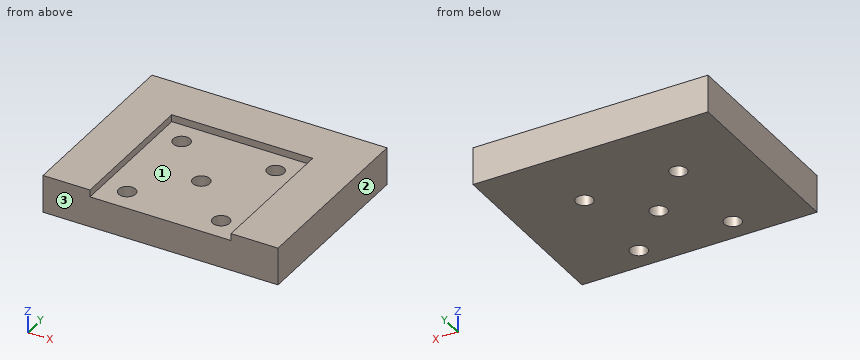
```python
from build123d import *
from build123d import SkipClean  # not in build123d's __all__

# Parameters (mm, degrees)
F0_R      = 2.85
F0_R_2    = 11
F1_DEPTH  = 40
F2_W      = 30
F2_H      = 30
F3_DEPTH  = 55
F5_DEPTH  = 30
F6_DEPTH  = 40.001
F7_DEPTH  = 40.001
F8_R      = 1.8
F9_DEPTH  = 11.5
F10_DEPTH = 13
F11_DEPTH = 5


with BuildPart() as f1:
    # F0 (on Front) → F1 (new body)
    with BuildSketch(Plane.XZ):
        with BuildLine():
            Line((15, 28.25), (-15, 28.25))
            ThreePointArc((-15, 28.25), (-22.0710678119, 25.3210678119), (-25, 18.25))
            Line((-25, 18.25), (-25, -38.25))
            Line((-25, -38.25), (25, -38.25))
            Line((25, -38.25), (25, 18.25))
            ThreePointArc((25, 18.25), (22.0710678119, 25.3210678119), (15, 28.25))
        make_face()
        with Locations((0, -18.25)):
            Circle(F0_R, mode=Mode.SUBTRACT)
        Circle(F0_R_2, mode=Mode.SUBTRACT)
        with Locations((0, 18.25)):
            Circle(F0_R, mode=Mode.SUBTRACT)
    extrude(amount=F1_DEPTH)

    # F2 (on face) → F3 (cut)
    with BuildSketch(Plane.XY.offset(28.25)):
        with Locations((0, -25)):
            Rectangle(F2_W, F2_H)
    extrude(amount=-F3_DEPTH, mode=Mode.SUBTRACT)

    # F4 (on face) → F5 (join, through all)
    with BuildSketch(Plane.XZ.offset(40)):
        with BuildLine():
            Line((-15, 17.2291616466), (-15, 19.972135955))
            ThreePointArc((-15, 19.972135955), (-20, 15.5), (-15, 11.027864045))
            Line((-15, 11.027864045), (-15, 13.7708383534))
            ThreePointArc((-15, 13.7708383534), (-17.3, 15.5), (-15, 17.2291616466))
        make_face()
        with BuildLine():
            Line((-15, -17.2291616466), (-15, -19.972135955))
            ThreePointArc((-15, -19.972135955), (-12.1458980338, -18.5), (-11, -15.5))
            ThreePointArc((-11, -15.5), (-12.1458980338, -12.5), (-15, -11.027864045))
            Line((-15, -11.027864045), (-15, -13.7708383534))
            ThreePointArc((-15, -13.7708383534), (-14.061250543, -14.4183346174), (-13.7, -15.5))
            ThreePointArc((-13.7, -15.5), (-14.061250543, -16.5816653826), (-15, -17.2291616466))
        make_face()
        with BuildLine():
            ThreePointArc((20, -15.5), (18.5, -12.1458980338), (15, -11.027864045))
            Line((15, -11.027864045), (15, -13.7708383534))
            ThreePointArc((15, -13.7708383534), (16.5816653826, -14.061250543), (17.3, -15.5))
            ThreePointArc((17.3, -15.5), (16.5816653826, -16.938749457), (15, -17.2291616466))
            Line((15, -17.2291616466), (15, -19.972135955))
            ThreePointArc((15, -19.972135955), (18.5, -18.8541019662), (20, -15.5))
        make_face()
        with BuildLine():
            Line((15, 17.2291616466), (15, 19.972135955))
            ThreePointArc((15, 19.972135955), (11, 15.5), (15, 11.027864045))
            Line((15, 11.027864045), (15, 13.7708383534))
            ThreePointArc((15, 13.7708383534), (13.7, 15.5), (15, 17.2291616466))
        make_face()
    extrude(amount=-F5_DEPTH)

    # F4 (on face) → F6 (cut, through all)
    with BuildSketch(Plane.XZ.offset(40)):
        with BuildLine():
            ThreePointArc((-13.7, 15.5), (-14.061250543, 16.5816653826), (-15, 17.2291616466))
            Line((-15, 17.2291616466), (-15, 13.7708383534))
            ThreePointArc((-15, 13.7708383534), (-14.061250543, 14.4183346174), (-13.7, 15.5))
        make_face()
        with BuildLine():
            ThreePointArc((17.3, 15.5), (16.5816653826, 16.938749457), (15, 17.2291616466))
            Line((15, 17.2291616466), (15, 13.7708383534))
            ThreePointArc((15, 13.7708383534), (16.5816653826, 14.061250543), (17.3, 15.5))
        make_face()
        with BuildLine():
            Line((15, -17.2291616466), (15, -13.7708383534))
            ThreePointArc((15, -13.7708383534), (13.7, -15.5), (15, -17.2291616466))
        make_face()
        with BuildLine():
            ThreePointArc((-15, -13.7708383534), (-17.3, -15.5), (-15, -17.2291616466))
            Line((-15, -17.2291616466), (-15, -13.7708383534))
        make_face()
    with SkipClean():  # cleaning this boolean's faces spoils the solid; the shape is the same uncleaned
        extrude(amount=-F6_DEPTH, mode=Mode.SUBTRACT)

    # F4 (on face) → F7 (cut, through all)
    with BuildSketch(Plane.XZ.offset(40)):
        with BuildLine():
            Line((-15, 13.7708383534), (-15, 17.2291616466))
            ThreePointArc((-15, 17.2291616466), (-17.3, 15.5), (-15, 13.7708383534))
        make_face()
        with BuildLine():
            Line((15, 13.7708383534), (15, 17.2291616466))
            ThreePointArc((15, 17.2291616466), (13.7, 15.5), (15, 13.7708383534))
        make_face()
        with BuildLine():
            Line((-15, -13.7708383534), (-15, -17.2291616466))
            ThreePointArc((-15, -17.2291616466), (-14.061250543, -16.5816653826), (-13.7, -15.5))
            ThreePointArc((-13.7, -15.5), (-14.061250543, -14.4183346174), (-15, -13.7708383534))
        make_face()
        with BuildLine():
            ThreePointArc((17.3, -15.5), (16.5816653826, -14.061250543), (15, -13.7708383534))
            Line((15, -13.7708383534), (15, -17.2291616466))
            ThreePointArc((15, -17.2291616466), (16.5816653826, -16.938749457), (17.3, -15.5))
        make_face()
    with SkipClean():  # cleaning this boolean's faces spoils the solid; the shape is the same uncleaned
        extrude(amount=-F7_DEPTH, mode=Mode.SUBTRACT)

    # F8 (on face) → F9 (cut, through all)
    with BuildSketch(Plane.XY.offset(-26.75)):
        with Locations((-10, -15)):
            Circle(F8_R)
        with Locations((10, -15)):
            Circle(F8_R)
        with Locations((-10, -35)):
            Circle(F8_R)
        with Locations((10, -35)):
            Circle(F8_R)
        with Locations((0, -25)):
            Circle(F8_R)
    extrude(amount=-F9_DEPTH, mode=Mode.SUBTRACT)

    # F10 (intersect): a face of the model
    f10_faces = [f1.faces().sort_by_distance(p)[0] for p in [
        (0, -19.8694432325, -38.25),
    ]]
    extrude(f10_faces, amount=-F10_DEPTH, mode=Mode.INTERSECT)

    # F11 (cut): a face of the model
    f11_faces = [f1.faces().sort_by_distance(p)[0] for p in [
        (0, -19.8694432325, -38.25),
    ]]
    extrude(f11_faces, amount=-F11_DEPTH, mode=Mode.SUBTRACT)


solid = f1.part
```
Part model, mm, in its own coordinate system. Face numbers are marked on the shaded views. Round coordinates to 2 decimals unless told otherwise and drop trailing zeros. Write each loop counter-clockwise with the first axis right and the second up, starting at its lowest first coordinate (ties: lowest second). Pieces come first, ordered by that corner, then holes. Notation, with made-up numbers: M -20,-37.75 L 30,-37.75 A9 ccw 30,-22.75 Z; hole C -38.5,-14 d11. An arc over 180 degrees is marked long. Answer as CSV lines item,"result". Start each with the question number.
1) Drop flat-ended pins along their axis: pin 1 (4.5 mm diameter, centred on x = 10, y = -35, fed in from +Z); pin 2 (2 mm diameter, centred on x = 10, y = -15, fed in from -Z). Give the stop position or say it passes through.
2) Band-saw the part on C-C (z = -31.25). List the corners of the cut face in (x, y).
3) Band-saw the part on D-D (x = 0). List the corners of the cut face in (y, z).
4) Band-saw the part on B-B (y = -25). List the corners of the cut face in (x, z).
5) Band-saw the part on A-A (x = -10). List the corners of the cut face in (y, z), then the cut area to 3 significant figures.
6) Mould opens along X. For the marked faces 1, 2 and 3 say: +X half, -X half, draft (parallel to the pull), parting line (faces both ways), or undercut.
7) Drill centre lines: L1, parallel to Y at x = 10, z = -28.75; L2, parallel to Y at x = 0, z = -30.5; L3, parallel to X at y = -12.5, z = -25.75. Where is each one in solid material? Low to high.
Worked out:
1,pin 1,"z = -26.75"
1,pin 2,"through"
2,outline,"M -25,-40 L 25,-40 L 25,0 L -25,0 Z; hole C -10,-35 d3.6; hole C -10,-15 d3.6; hole C 0,-25 d3.6; hole C 10,-35 d3.6; hole C 10,-15 d3.6"
3,outline,"M -40,-33.25 L -26.8,-33.25 L -26.8,-26.75 L -40,-26.75 Z; M -23.2,-33.25 L 0,-33.25 L 0,-25.25 L -10,-25.25 L -10,-26.75 L -23.2,-26.75 Z"
4,outline,"M -25,-33.25 L -1.8,-33.25 L -1.8,-26.75 L -15,-26.75 L -15,-25.25 L -25,-25.25 Z; M 1.8,-33.25 L 25,-33.25 L 25,-25.25 L 15,-25.25 L 15,-26.75 L 1.8,-26.75 Z"
5,outline,"M -40,-33.25 L -36.8,-33.25 L -36.8,-26.75 L -40,-26.75 Z; M -33.2,-33.25 L -16.8,-33.25 L -16.8,-26.75 L -33.2,-26.75 Z; M -13.2,-33.25 L 0,-33.25 L 0,-25.25 L -10,-25.25 L -10,-26.75 L -13.2,-26.75 Z"
5,area,"228 mm²"
6,face 1,"undercut"
6,face 2,"+X half"
6,face 3,"draft"
7,L1,"-40 to -36.8, -33.2 to -16.8, -13.2 to 0"
7,L2,"-40 to -26.8, -23.2 to 0"
7,L3,"-25 to -15, 15 to 25"
